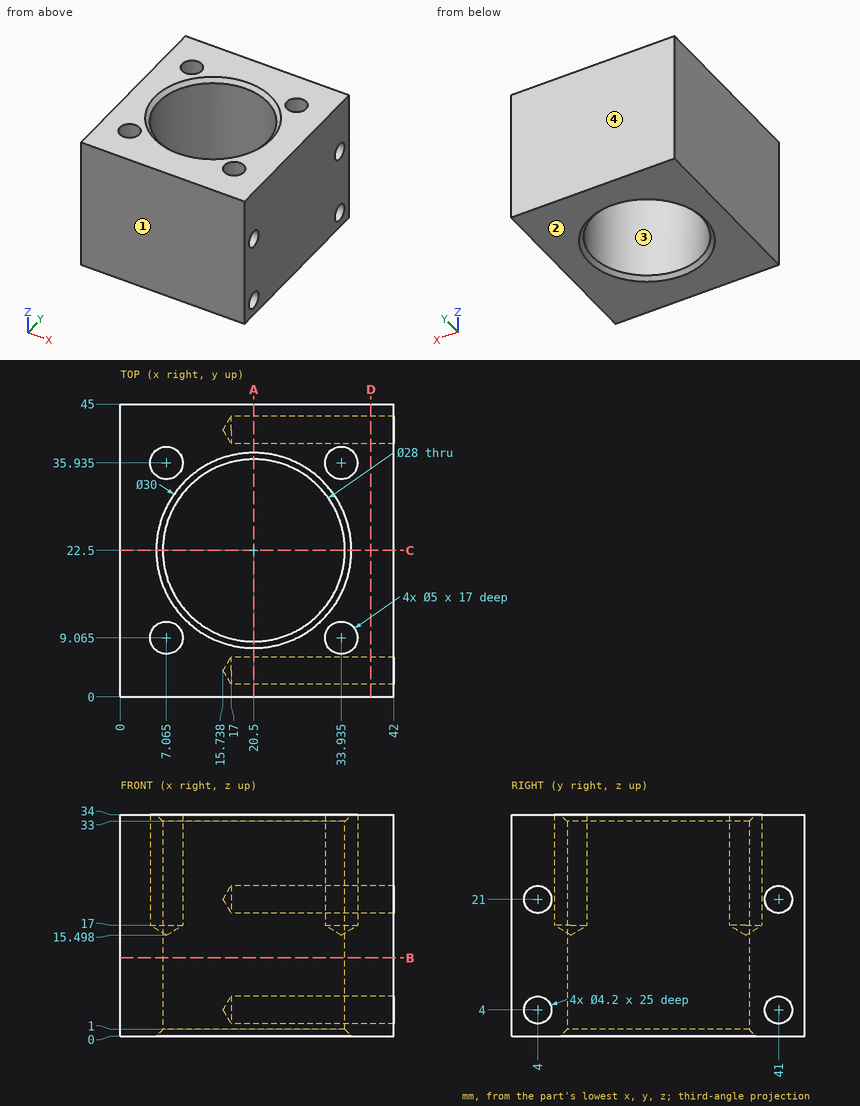
For this review, use the dimensioned drawing (mm, ordinates from the lowest corner) and the shaded views. Give positions to 0.01 mm unless a question says otherwise; leave off trailing zeros. Order: outer loops, then holes, each group sorted by start corner. A loop starts at its lowest first (then second) coordinate and runs counter-clockwise, first axis right, second up.
1) The part is to be moulded in two halves that separate along Y. For the marked faces 1, 2, 3 and 4, say which applies: released by +Y, released by -Y, zero draft, split by the parting line, or undercut.
2) Take a section at A-A (x = 20.5). Give the boundary of the cut face in (y, z).
3) Take a section at C-C (y = 22.5). Give the boundary of the cut face in (x, z).
4) Insertion check: pin 1 (3 mm diameter, centred on x = 7.06, y = 9.06, fed in from +Z). The pin has a flat end and moves straight along its axis. Give the tip position at first contact, or say it passes through.
5) Take a section at B-B (z = 12). Give the boundary of the cut face in (x, y).
6) Take a section at D-D (x = 38.5). Give the boundary of the cut face in (y, z).
7) Wall thickness on line 1 (Y direction, x = 36, z = 4); line 2 (Z direction, x = 23, y = 41); line 3 (Y direction, x = 24, z = 4) (1 decimal): over which ranges is each line inside the solid? List them lowest first.
Derived:
1. face 1: released by -Y
1. face 2: zero draft
1. face 3: undercut
1. face 4: released by +Y
2. outline: (0, 0) - (7.5, 0) - (8.5, 1) - (8.5, 33) - (7.5, 34) - (0, 34) - close; (36.5, 1) - (37.5, 0) - (45, 0) - (45, 34) - (37.5, 34) - (36.5, 33) - close; hole circle Ø4.2 at (4, 4); hole circle Ø4.2 at (4, 21); hole circle Ø4.2 at (41, 4); hole circle Ø4.2 at (41, 21)
3. outline: (0, 0) - (5.5, 0) - (6.5, 1) - (6.5, 33) - (5.5, 34) - (0, 34) - close; (34.5, 1) - (35.5, 0) - (42, 0) - (42, 34) - (35.5, 34) - (34.5, 33) - close
4. pin 1: stops at z = 16.4
5. outline: (0, 0) - (42, 0) - (42, 45) - (0, 45) - close; hole circle Ø28 at (20.5, 22.5)
6. outline: (0, 0) - (45, 0) - (45, 34) - (0, 34) - close; hole circle Ø4.2 at (4, 4); hole circle Ø4.2 at (4, 21); hole circle Ø4.2 at (41, 4); hole circle Ø4.2 at (41, 21)
7. line 1: y = 0 to 1.9, 6.1 to 38.9, 43.1 to 45
7. line 2: z = 0 to 1.9, 6.1 to 18.9, 23.1 to 34
7. line 3: y = 0 to 1.9, 6.1 to 8.9, 36.1 to 38.9, 43.1 to 45
